Could you check a few things on this model? Use its own coordinates, in mm. A direction names the side the tool comes from. Give positions to 0.01 mm unless a question says otherwise; leave off trailing zeros. Loops run counter-clockwise (first coordinate to the right, second up) from the corner with the lowest first, then second, coordinate; pieces in that order, holes last. Notation, with made-up numbers: (74.5, -18.5) - (126.5, -18.5) arc R13 ccw to (126.5, -9.5) - close; hole circle Ø8 at (27.25, 77). An arc over 180 degrees is marked (long way). Write each question's results on one line, items separated by ' | '. Start each with the question number.
1) If I drill on probe 1 along Z at (x, y) = (-15.5, -20); probe 2 along Y at (x, z) = (16, 6); probe 3 along X at (y, z) = (-14, -2), over which ranges is the centre line in solid material (lowest first)? Write a range as [from, to].
2) If we mould it in two halves opening along Z, with no side actions, what happens to faces 1 (the face through (-1, -18, 12.7)), 2 (the face through (-96.461, -6, 0)), 3 (the face through (-1, -25, -19.05))? For each: +Z half, -Z half, draft (parallel to the pull), parting line (faces both ways), or undercut.
3) I want a section at D-D, the plane z = -15.5. Write out the boundary of the cut face in (x, y).
4) I want a section at A-A, the plane z = -4.5. Write out the boundary of the cut face in (x, y), and give its area (3 significant figures).
5) I want a section at C-C, the plane y = -7.5. Write out the boundary of the cut face in (x, z).
6) I'm going to push flat-ended pins straight in: pin 1 (1 mm diameter, centred on y = -23.5, z = -2.5, fed in from -X); pin 2 (7.5 mm diameter, centred on y = -19.5, z = 3, fed in from +X); pin 3 (1.5 mm diameter, centred on y = -20.5, z = -13, fed in from +X). Where does each tip first touch, or does it pass through?
7) I want a section at B-B, the plane x = 29.5. Write out the boundary of the cut face in (y, z), and give its area (3 significant figures).
8) On a 3-axis mill with a long thin cutter (end or side, diameter ignored), from which of +Z, -Z, +X, -X, +Y, -Y can I reach the whole of each face in a straight line? I mean faces 4 (the face through (-1, -35.56, 0)), 5 (the face through (-77.47, -16, 0)), 6 (the face through (81.38, -27.78, 0.27)), 7 (the face through (-1, -25, 19.05)), 8 (the face through (-1, -18, -12.7)). Say none if no direction works.
from build123d import *

# Parameters (mm, degrees)
SKETCH1_W           = 192.921126566
SKETCH1_H           = 38.1
SKETCH1_W_2         = 154.94
SKETCH1_H_2         = 25.4
BOSS_EXTRUDE4_DEPTH = 50.8
CHAMFER2_SIZE       = 38.1
SKETCH1_5_W         = 154.94
SKETCH1_5_H         = 25.4
CUT_EXTRUDE1_DEPTH  = 35.56


with BuildPart() as part:
    # Sketch1 → Boss-Extrude4 (new body)
    # profile 1 of 2: a face of its own
    with BuildSketch(Plane(origin=(0, 0, 0), x_dir=(1, 0, 0), z_dir=(0, 1, 0))):
        Rectangle(SKETCH1_W, SKETCH1_H)
        Rectangle(SKETCH1_W_2, SKETCH1_H_2, mode=Mode.SUBTRACT)
    # profile 2 of 2: a face of its own
    with BuildSketch(Plane(origin=(0, 0, 0), x_dir=(1, 0, 0), z_dir=(0, 1, 0))):
        Rectangle(SKETCH1_W_2, SKETCH1_H_2)
    extrude(amount=-BOSS_EXTRUDE4_DEPTH)

    # Chamfer2
    chamfer2_edges = [part.edges().sort_by_distance(p)[0] for p in [
        (96.460563283, -50.8, 0),
        (-96.460563283, -50.8, 0),
    ]]
    chamfer(chamfer2_edges, length=CHAMFER2_SIZE)

    # Sketch1_5 → Cut-Extrude1 (cut)
    with BuildSketch(Plane(origin=(0, 0, 0), x_dir=(1, 0, 0), z_dir=(0, 1, 0))):
        Rectangle(SKETCH1_5_W, SKETCH1_5_H)
    extrude(amount=-CUT_EXTRUDE1_DEPTH, mode=Mode.SUBTRACT)


solid = part.part
Answers:
1) probe 1: z = [-19.05, -12.7], [12.7, 19.05] | probe 2: y = [-50.8, -35.56] | probe 3: x = [-95.16, -77.47], [77.47, 95.16]
2) face 1: undercut | face 2: draft | face 3: -Z half
3) outline: (-96.46, -12.7) - (-58.36, -50.8) - (58.36, -50.8) - (96.46, -12.7) - (96.46, 0) - (-96.46, 0) - close
4) outline: (-96.46, -12.7) - (-77.47, -31.69) - (-77.47, 0) - (-96.46, 0) - close; (-73.6, -35.56) - (-58.36, -50.8) - (58.36, -50.8) - (73.6, -35.56) - close; (77.47, -31.69) - (96.46, -12.7) - (96.46, 0) - (77.47, 0) - close | area: 2,850 mm2
5) outline: (-96.46, -19.05) - (96.46, -19.05) - (96.46, 19.05) - (-96.46, 19.05) - close; hole (-77.47, -12.7) - (77.47, -12.7) - (77.47, 12.7) - (-77.47, 12.7) - close
6) pin 1: stops at x = -86.16 | pin 2: stops at x = 93.41 | pin 3: stops at x = 89.41
7) outline: (-50.8, -19.05) - (0, -19.05) - (0, -12.7) - (-35.56, -12.7) - (-35.56, 12.7) - (0, 12.7) - (0, 19.05) - (-50.8, 19.05) - close | area: 1,030 mm2
8) face 4: +X, -X, +Y | face 5: +Y, -Y | face 6: +Z, -Z, +X, -Y | face 7: +Z, +X, -X, +Y, -Y | face 8: +Y
